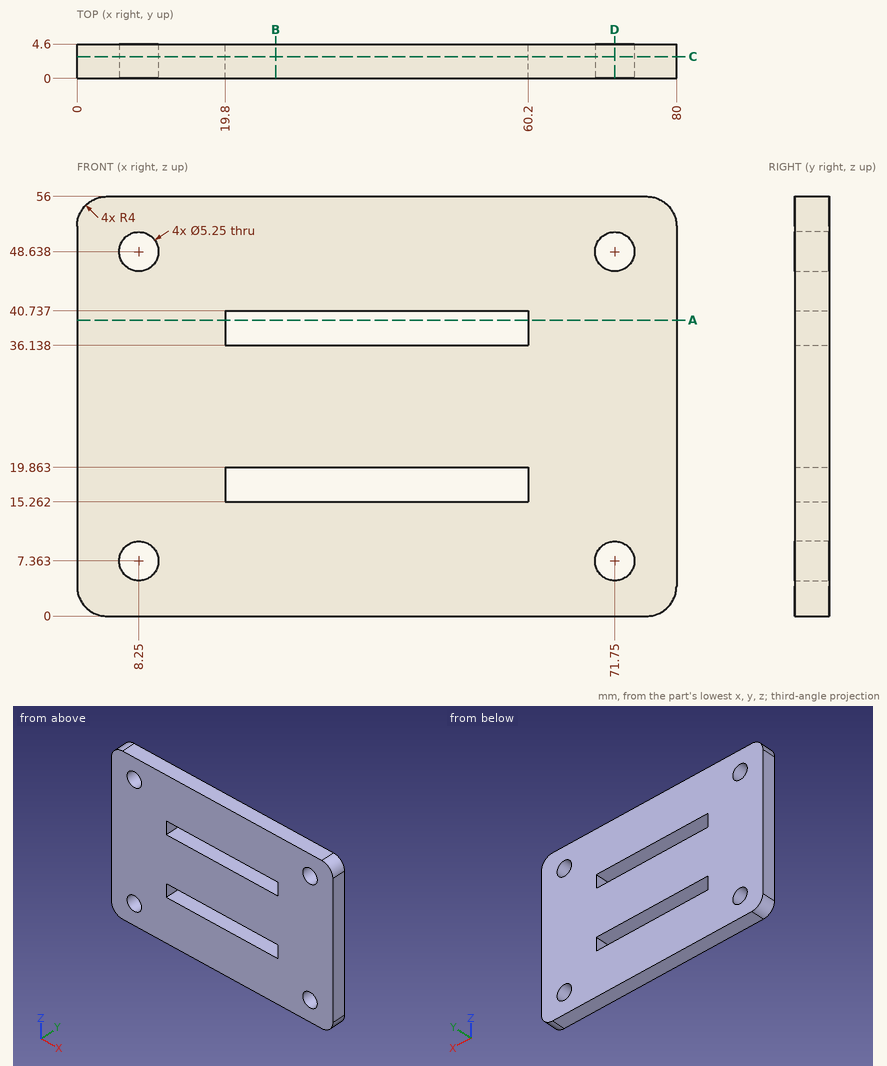
Answer from the drawing. Dimensions are ordinates in mm from the lowest x, y and z of the part. Give positions to 0.01 mm unless a question says otherwise; leave off trailing zeros. Order: outer loops, then holes, each group sorted by start corner. A loop starts at its lowest first (then second) coordinate and runs counter-clockwise, first axis right, second up.
Item 1: Find the intervals of material crossed by probe 1 along Z at (x, y) = (71.75, 1.95); probe 2 along Z at (x, y) = (32.5, 0.55); probe 3 along X at (y, z) = (0.7, 16.5), in increasing order.
From the geometry:
probe 1: z = 0 to 4.74, 9.99 to 46.01, 51.26 to 56
probe 2: z = 0 to 15.26, 19.86 to 36.14, 40.74 to 56
probe 3: x = 0 to 19.8, 60.2 to 80
Item 2: Given pin 1 Ø3 at (x, z) = (71.75, 48.64) entering from +Y, flat-ended and moving along its own axis, determine where the tip first touches the part or whether it passes through.
From the geometry:
pin 1: passes through
Item 3: The part is cut by section C-C, the plane y = 2.9. Count the separate pieces of the cut face and the enclosed holes in it, and give its area (3 significant figures).
From the geometry:
separate pieces: 1
enclosed holes: 6
area: 4,010 mm2
Item 4: The part is cut by section D-D, the plane x = 71.75. Give the vertices of the cut face in (y, z).
From the geometry:
outline: (0, 0) - (4.6, 0) - (4.6, 4.74) - (0, 4.74) - close; (0, 9.99) - (4.6, 9.99) - (4.6, 46.01) - (0, 46.01) - close; (0, 51.26) - (4.6, 51.26) - (4.6, 56) - (0, 56) - close
Item 5: The part is cut by section A-A, the plane z = 39.5. Give the vertices of the cut face in (x, y), and give its area (3 significant figures).
From the geometry:
outline: (0, 0) - (19.8, 0) - (19.8, 4.6) - (0, 4.6) - close; (60.2, 0) - (80, 0) - (80, 4.6) - (60.2, 4.6) - close
area: 182 mm2
Item 6: The part is cut by section B-B, the plane x = 26.5. Give the vertices of the cut face in (y, z).
From the geometry:
outline: (0, 0) - (4.6, 0) - (4.6, 15.26) - (0, 15.26) - close; (0, 19.86) - (4.6, 19.86) - (4.6, 36.14) - (0, 36.14) - close; (0, 40.74) - (4.6, 40.74) - (4.6, 56) - (0, 56) - close
